Model file for the job. Use its own axes, mm. Face numbers are marked on the shaded views. A direction names the side the tool comes from. Coordinates: 2 decimals unless noted, no trailing zeros. Loops run counter-clockwise (first coordinate to the right, second up) from the corner with the lowest first, then second, coordinate; pieces in that order, holes last.
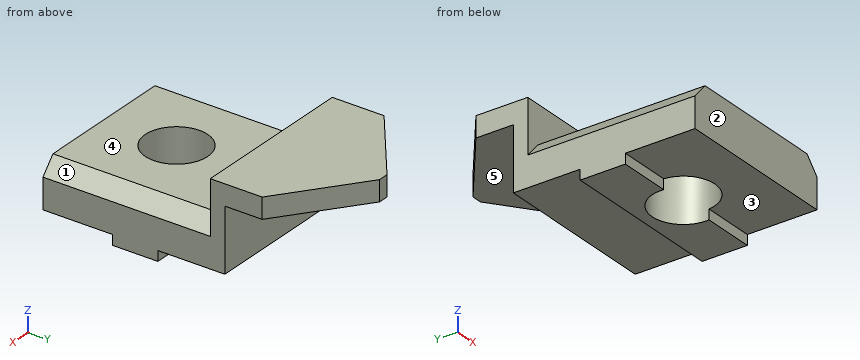
from build123d import *

# Parameters (mm, degrees)
F0_W      = 76.2
F0_H      = 76.2
F1_DEPTH  = 25.4
F0_H_2    = 50.8
F2_DEPTH  = 42.672
F4_DEPTH  = 76.2
F5_R      = 14.224
F6_DEPTH  = 25.4
F7_W      = 31.75
F7_H      = 4.572
F7_W_2    = 74.676
F8_DEPTH  = 96.266
F10_W     = 76.2
F10_H     = 28.702
F11_DEPTH = 44.196
F12_DEPTH = 25.4


with BuildPart() as f1:
    # F0 (on Top) → F1 (new body)
    with BuildSketch(Plane.XY):
        with Locations((2.621409, -8.470273)):
            Rectangle(F0_W, F0_H)
    extrude(amount=F1_DEPTH)

    # F0 (on Top) → F2 (join)
    with BuildSketch(Plane.XY):
        with Locations((2.621409, 55.029727)):
            Rectangle(F0_W, F0_H_2)
    extrude(amount=F2_DEPTH)

    # F3 (on face) → F4 (cut)
    with BuildSketch(Plane.XZ.offset(46.570273)):
        Polygon((40.721409, 25.4), (34.48936, 25.4), (40.721409, 18.365515), align=None)
        Polygon((-35.478591, 18.365515), (-29.246543, 25.4), (-35.478591, 25.4), align=None)
    extrude(amount=-F4_DEPTH, mode=Mode.SUBTRACT)

    # F5 (on face) → F6 (cut)
    with BuildSketch(Plane.XY.offset(25.4)):
        with Locations((2.621409, -13.519656)):
            Circle(F5_R)
    extrude(amount=-F6_DEPTH, mode=Mode.SUBTRACT)

    # F7 (on face) → F8 (cut)
    with BuildSketch(Plane.YZ.offset(40.721409)):
        with Locations((-30.695273, 2.286)):
            Rectangle(F7_W, F7_H)
        with Locations((43.091727, 2.286)):
            Rectangle(F7_W_2, F7_H)
    extrude(amount=-F8_DEPTH, mode=Mode.SUBTRACT)

    # F10 (on face) → F11 (cut)
    with BuildSketch(Plane(origin=(0, 80.429727, 0), x_dir=(-1, 0, 0), z_dir=(0, 1, 0))):
        with Locations((-2.621409, 18.923)):
            Rectangle(F10_W, F10_H)
    extrude(amount=-F11_DEPTH, mode=Mode.SUBTRACT)

    # F9 (on face) → F12 (cut)
    with BuildSketch(Plane.XY.offset(42.672)):
        Polygon((4.572, 80.429727), (40.721409, 53.251727), (40.721409, 80.429727), align=None)
        Polygon((-35.478591, 80.429727), (-35.478591, 53.251727), (0, 80.429727), align=None)
    extrude(amount=-F12_DEPTH, mode=Mode.SUBTRACT)


solid = f1.part
Q1. Flat gauge pins, fed straight in: P1, Ø16, axis at x = 0, y = -38.5, coming from the -Z side; P2, Ø3.5, axis at x = -19.5, z = 2, coming from the -Y side; P3, Ø6, axis at x = -24, y = 25.5, coming from the +Z side; P4, Ø8, axis at x = 32.5, y = 26.5, coming from the +Z side. Where does each tip first touch, or does it go through?
Answers:
P1: stops at z = 4.57
P2: stops at y = -14.82
P3: stops at z = 25.4
P4: stops at z = 42.67
Q2. Slice it at A-A (z = 17). List the corners of the cut face in (x, y), and give its area (3 significant figures).
Answers:
outline: (-35.48, -46.57) - (40.72, -46.57) - (40.72, 36.23) - (-35.48, 36.23) - close; hole circle Ø28.45 at (2.62, -13.52)
area: 5,670 mm2
Q3. Slice it at C-C (y = 47). List the corners of the cut face in (x, z).
Answers:
outline: (-35.48, 33.27) - (40.72, 33.27) - (40.72, 42.67) - (-35.48, 42.67) - close
Q4. Drill centre lines: line 1 (Z direction, x = -20.5, y = 52); line 2 (Z direction, x = 33.5, y = 5.5); line 3 (Y direction, x = -11, z = 33). Where is each one in solid material? Low to high.
Answers:
line 1: z = 33.27 to 42.67
line 2: z = 0 to 25.4
line 3: y = 29.63 to 36.23
Q5. Slice it at B-B (x = -10). List the corners of the cut face in (y, z), and give its area (3 significant figures).
Answers:
outline: (-46.57, 4.57) - (-20.08, 4.57) - (-20.08, 25.4) - (-46.57, 25.4) - close; (-6.96, 0) - (5.75, 0) - (5.75, 4.57) - (36.23, 4.57) - (36.23, 33.27) - (72.77, 33.27) - (72.77, 42.67) - (29.63, 42.67) - (29.63, 25.4) - (-6.96, 25.4) - close
area: 1,970 mm2
Q6. Slice it at D-D (z = 35.5). List the corners of the cut face in (x, y), and give its area (3 significant figures).
Answers:
outline: (-35.48, 29.63) - (40.72, 29.63) - (40.72, 53.25) - (4.57, 80.43) - (0, 80.43) - (-35.48, 53.25) - close
area: 2,900 mm2
Q7. Which spindle directions (+Z, -Z, +X, -X, +Y, -Y) get a long thin tool onto all of the face, cutting with end or side? Do the marked faces 1, 2, 3, 4 and 5. Say none if no direction does.
Answers:
face 1: +Z, +X, -Y
face 2: +Z, -Z, +X, -X, -Y
face 3: -Z, +X, -X, -Y
face 4: +Z, +X, -X, -Y
face 5: -Z, +X, -X, +Y
